```python
from build123d import *

# Parameters (mm, degrees)
BOSS_EXTRUDE1_DEPTH = 4
CIRPATTERN1_COUNT   = 5


with BuildPart() as part:
    # Sketch1 → Revolve1 (revolve)
    with BuildSketch(Plane(origin=(0, 0, 0), x_dir=(0, 0, -1), z_dir=(1, 0, 0)), mode=Mode.PRIVATE) as revolve1_sk:
        Polygon((0, 0), (29.164360148, 0), (29.5, -0.4), (26.2, -1.9), (26.2, -0.9), (22.1, -0.9), (22.1, -1.9), (0, -1.9), align=None)
    revolve(revolve1_sk.sketch.rotate(Axis((0, 64.33779776, 0), (0, -1, 0)), 180), axis=Axis((0, 64.33779776, 0), (0, -1, 0)))

    # Sketch2 → Boss-Extrude1 (add)
    with BuildSketch(Plane.XZ.offset(1.9)):
        with BuildLine():
            Line((9.35, 18.243560508), (3.85, 13.033927997))
            ThreePointArc((3.85, 13.033927997), (0, 11.5), (-3.85, 13.033927997))
            Line((-3.85, 13.033927997), (-9.35, 18.243560508))
            ThreePointArc((-9.35, 18.243560508), (0, 20.5), (9.35, 18.243560508))
        make_face()
    boss_extrude1 = extrude(amount=BOSS_EXTRUDE1_DEPTH)

    # CirPattern1: Boss-Extrude1 ×5 about axis
    cirpattern1_axis = Axis((0, 0, 0), (0, 1, 0))
    for i in range(1, CIRPATTERN1_COUNT):
        add(boss_extrude1.rotate(cirpattern1_axis, i * 360 / CIRPATTERN1_COUNT))


solid = part.part
```
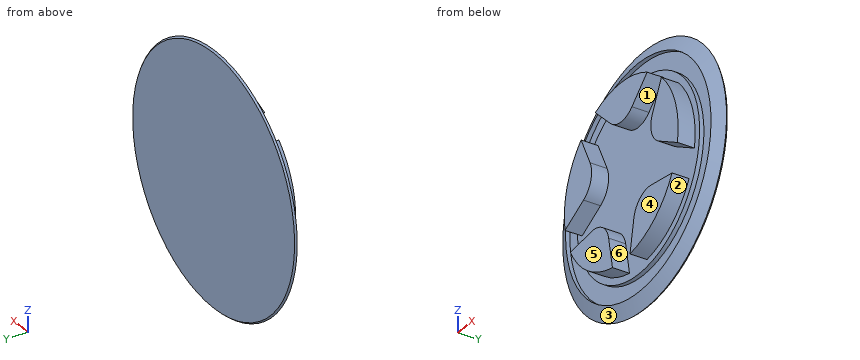
Here's how the part is built. I have some questions about the finished solid (model axes, mm). Face numbers are marked on the shaded views. A direction names the side the tool comes from. Round coordinates to 2 decimals unless told otherwise and drop trailing zeros. Order: outer loops, then holes, each group sorted by start corner. A loop starts at its lowest first (then second) coordinate and runs counter-clockwise, first axis right, second up. Notation, with made-up numbers: (63.25, -27) -> (74.25, -27) arc R16 ccw to (74.25, -13) -> close; hole circle Ø8 at (40, 83). An arc over 180 degrees is marked (long way). Use a Markdown table: item, result. Add a question column.
(1) Suppose I cut it at A-A, the plane y = -3.8. Please give me the cut outline in (x, z), and give its area (3 significant figures).
(2) For pin 1 Ø2 at (x, z) = (8.5, 11.5) entering from -Y, with a flat end and sliding along its axis, tell me the tip position at first contact or that it passes through.
(3) If we mould it in two halves opening along X, with no side actions, what happens to the marked faces 1, 2, 3 and 4? For each: released by +X, released by -X, zero draft, split by the parting line, or undercut.
(4) I need wall thicknesses on line 1 along X through (y, z) = (-3.25, 14); line 2 along X through (y, z) = (-1.65, 0); line 3 along Y through (x, z) = (25.5, 1). Which ranges of each line are inside material? Lowest first, please.
(5) For the marked faces 5 and 6, which set-ups out of +Z, -Z, +X, -X, +Y, -Y let a thin tool reach every point of the face, with its end or its side?
(6) Suppose I cut it at B-B, the plane x = 0. Please give me the cut outline in (y, z).
Verdict:
| question | item | result |
|---|---|---|
| 1 | outline | (-20.24, -3.25) -> (-13.59, 0.37) arc R5.6 ccw to (-11.21, 7.69) -> (-14.46, 14.53) arc R20.5 ccw to start; (-18.29, -9.26) arc R20.5 ccw to (-3.16, -20.26) -> (-4.55, -12.81) arc R5.6 ccw to (-10.78, -8.28) -> close; (-9.35, 18.24) -> (-3.85, 13.03) arc R5.6 ccw to (3.85, 13.03) -> (9.35, 18.24) arc R20.5 ccw to start; (3.16, -20.26) arc R20.5 ccw to (18.29, -9.26) -> (10.78, -8.28) arc R5.6 ccw to (4.55, -12.81) -> close; (11.21, 7.69) arc R5.6 ccw to (13.59, 0.37) -> (20.24, -3.25) arc R20.5 ccw to (14.46, 14.53) -> close |
| 1 | area | 527 mm2 |
| 2 | pin 1 | y = -1.9 |
| 3 | face 1 | undercut |
| 3 | face 2 | released by +X |
| 3 | face 3 | split by the parting line |
| 3 | face 4 | zero draft |
| 4 | line 1 | -14.97 to -14.21, -4.87 to 4.87, 14.21 to 14.97 |
| 4 | line 2 | -26.75 to -26.2, -22.1 to 22.1, 26.2 to 26.75 |
| 4 | line 3 | -0.9 to 0 |
| 5 | face 5 | +Z, -Z, +X, -X, -Y |
| 5 | face 6 | -Y |
| 6 | outline | (-5.9, 11.5) -> (-1.9, 11.5) -> (-1.9, -22.1) -> (-0.9, -22.1) -> (-0.9, -26.2) -> (-1.9, -26.2) -> (-0.4, -29.5) -> (0, -29.16) -> (0, 29.16) -> (-0.4, 29.5) -> (-1.9, 26.2) -> (-0.9, 26.2) -> (-0.9, 22.1) -> (-1.9, 22.1) -> (-1.9, 20.5) -> (-5.9, 20.5) -> close |
